from build123d import *

# Parameters (mm, degrees)
BASE_FLANGE3_DEPTH = 406.4
SKETCH10_R         = 1.4478
CUT_EXTRUDE3_DEPTH = 594.198769469
SKETCH11_R         = 2.032
CUT_EXTRUDE4_DEPTH = 594.139546967


# Sheet-metal steps are written as plain solids
with BuildPart() as part:
    # Sketch1 → Base-Flange3 (new body)
    with BuildSketch(Plane.XY):
        with BuildLine():
            Line((431.8, 16.51), (431.8, 2.4384))
            ThreePointArc((431.8, 2.4384), (431.085809175, 0.714190825), (429.3616, 0))
            Line((429.3616, 0), (2.4384, 0))
            ThreePointArc((2.4384, 0), (0.714190825, 0.714190825), (0, 2.4384))
            Line((0, 2.4384), (0, 16.51))
            Line((0, 16.51), (2.286, 16.51))
            Line((2.286, 16.51), (2.286, 2.4384))
            ThreePointArc((2.286, 2.4384), (2.330636927, 2.330636927), (2.4384, 2.286))
            Line((2.4384, 2.286), (429.3616, 2.286))
            ThreePointArc((429.3616, 2.286), (429.469363073, 2.330636927), (429.514, 2.4384))
            Line((429.514, 2.4384), (429.514, 16.51))
            Line((429.514, 16.51), (431.8, 16.51))
        make_face()
    extrude(amount=BASE_FLANGE3_DEPTH)

    # Sketch10 → Cut-Extrude3 (cut, through all)
    with BuildSketch(Plane(origin=(431.8, 0, 0), x_dir=(0, 0, -1), z_dir=(1, 0, 0))):
        with Locations((-31.75, 10.16)):
            Circle(SKETCH10_R)
        with Locations((-146.05, 10.16)):
            Circle(SKETCH10_R)
        with Locations((-260.35, 10.16)):
            Circle(SKETCH10_R)
        with Locations((-374.65, 10.16)):
            Circle(SKETCH10_R)
    extrude(amount=-CUT_EXTRUDE3_DEPTH, mode=Mode.SUBTRACT)

    # Sketch11 → Cut-Extrude4 (cut, through all)
    with BuildSketch(Plane(origin=(0, 2.286, 0), x_dir=(-1, 0, 0), z_dir=(0, 1, 0))):
        with Locations(Location((-406.4, 397.002, 0), (0, 0, 90))):
            Circle(SKETCH11_R)
        with Locations(Location((-279.4, 397.002, 0), (0, 0, 90))):
            Circle(SKETCH11_R)
        with Locations(Location((-152.4, 397.002, 0), (0, 0, 90))):
            Circle(SKETCH11_R)
        with Locations(Location((-25.4, 397.002, 0), (0, 0, 90))):
            Circle(SKETCH11_R)
        with Locations(Location((-406.4, 9.398, 0), (0, 0, 90))):
            Circle(SKETCH11_R)
        with Locations(Location((-279.4, 9.398, 0), (0, 0, 90))):
            Circle(SKETCH11_R)
        with Locations(Location((-152.4, 9.398, 0), (0, 0, 90))):
            Circle(SKETCH11_R)
        with Locations(Location((-25.4, 9.398, 0), (0, 0, 90))):
            Circle(SKETCH11_R)
    extrude(amount=-CUT_EXTRUDE4_DEPTH, mode=Mode.SUBTRACT)


solid = part.part
Geometry: final body of the model. Coordinates: model frame, mm. A direction names the side the tool comes from. Round coordinates to 2 decimals unless told otherwise and drop trailing zeros. Order: outer loops, then holes, each group sorted by start corner. A loop starts at its lowest first (then second) coordinate and runs counter-clockwise, first axis right, second up.
Q1. Access query for faces 1 (the face through (2.286, 10, 200)), 2 (the face through (217, 2, 0)). Directions: +Z, -Z, +X, -X, +Y, -Y. A direction counts if a zero-diameter tool reaches every point of the face in a straight line with its end or side. Return the directions, or none.
Result sheet:
face 1: +Z, -Z, +Y
face 2: -Z, +X, -X, +Y, -Y
Q2. Section B-B, the plane x = 76.5. Output: boundary loops of the cut face in (y, z), and give its area (3 significant figures).
Result sheet:
outline: (0, 0) - (2.29, 0) - (2.29, 406.4) - (0, 406.4) - close
area: 929 mm2
Q3. Section A-A, the plane z = 349. Output: boundary loops of the cut face in (x, y).
Result sheet:
outline: (0, 2.44) arc R2.44 ccw to (2.44, 0) - (429.36, 0) arc R2.44 ccw to (431.8, 2.44) - (431.8, 16.51) - (429.51, 16.51) - (429.51, 2.44) arc R0.15 cw to (429.36, 2.29) - (2.44, 2.29) arc R0.15 cw to (2.29, 2.44) - (2.29, 16.51) - (0, 16.51) - close
Q4. Pin query (flat end, axial travel): pin 1 (6 mm diameter, centred on x = 176.5, z = 236.5, fed in from +Y). Return the tip coordinate at first contact, or that it passes through.
Result sheet:
pin 1: stops at y = 2.29
Q5. Material intervals for probe 1 along X at (y, z) = (12, 261); probe 2 along Y at (x, z) = (171, 224); probe 3 along X at (y, z) = (2, 265.5), sorted ascending.
Result sheet:
probe 1: x = 0 to 2.29, 429.51 to 431.8
probe 2: y = 0 to 2.29
probe 3: x = 0.04 to 431.76
